CAD build for the part. Positions are in the model's coordinates, mm. A direction names the side the tool comes from. Give positions to 0.01 mm unless a question says otherwise; leave off trailing zeros. Write each loop counter-clockwise with the first axis right and the second up, starting at its lowest first coordinate (ties: lowest second). Pieces come first, ordered by that corner, then holes. Notation, with made-up numbers: (14.5, 22.25) - (70.5, 22.25) arc R18 ccw to (70.5, 50.25) - close; hole circle Ø10 at (79.5, -10). An arc over 180 degrees is marked (long way). Answer as a JSON object with one key per item and string values.
Autodesk Inventor part; units mm, degrees
ref_plane "YZ Plane" through (0, 0, 0) normal (1, 0, 0) x (0, 1, 0)
ref_plane "XZ Plane" through (0, 0, 0) normal (0, 1, 0) x (-1, 0, 0)
ref_plane "XY Plane" through (0, 0, 0) normal (0, 0, 1) x (1, 0, 0)
sketch "Sketch2" plane through (0, 0, 0) normal (0, 1, 0) x (-1, 0, 0)
  line L0 (0, 0) -> (85, 0)
  line L1 (85, 0) -> (85, -25)
  line L2 (85, -25) -> (0, -25)
  line L3 (0, -25) -> (0, 0)
  line L4 (-5, -25) -> (105, -25)
  line L5 (105, -25) -> (105, -40)
  line L6 (105, -40) -> (-5, -40)
  line L7 (-5, -40) -> (-5, -25)
  line L8 (-5, -25) -> (0, -20)
  dimension "d4" = 85
  dimension "d5" = 25
  dimension "d6" = 110
  dimension "d7" = 5
  dimension "d8" = 15
  dimension "d9" = 45
extrude "Extrusion2" add sketch "Sketch2" along normal blind 88
sketch "Sketch3" plane through (-105, 0, -25) normal (0, 0, 1) x (1, 0, 0)
  line L0 (20, 0) -> (20, 88)
  line L1 (20, 83) -> (1, 83)
  line L2 (1, 83) -> (1, 33)
  line L3 (1, 33) -> (20, 33)
  line L4 (20, 33) -> (20, 83)
  line L5 (0, 88) -> (20, 88)
  point P0 (105, 0)
  point P1 (20, 33)
  dimension "d12" = 50
  dimension "d13" = 19
  dimension "d14" = 5
extrude "Extrusion3" add sketch "Sketch3" along normal blind 15
sketch "Sketch4" plane through (-104, 33, -25) normal (-1, 0, 0) x (0, 0, 1)
  line L0 (6, 7.5) -> (11, 7.5)
  line L1 (11, 7.5) -> (11, 2.5)
  line L2 (11, 2.5) -> (6, 2.5)
  line L3 (6, 2.5) -> (6, 7.5)
  line L4 (0, -33) -> (0, 55)
  line L5 (0, 0) -> (15, 0)
  line L6 (6, 17.5) -> (11, 17.5)
  line L7 (11, 17.5) -> (11, 12.5)
  line L8 (6, 12.5) -> (6, 17.5)
  line L9 (11, 12.5) -> (6, 12.5)
  line L10 (6, 27.5) -> (11, 27.5)
  line L11 (11, 27.5) -> (11, 22.5)
  line L12 (6, 22.5) -> (6, 27.5)
  line L13 (11, 22.5) -> (6, 22.5)
  line L14 (6, 37.5) -> (11, 37.5)
  line L15 (11, 37.5) -> (11, 32.5)
  line L16 (6, 32.5) -> (6, 37.5)
  line L17 (11, 32.5) -> (6, 32.5)
  line L18 (6, 47.5) -> (11, 47.5)
  line L19 (11, 47.5) -> (11, 42.5)
  line L20 (6, 42.5) -> (6, 47.5)
  line L21 (11, 42.5) -> (6, 42.5)
  point P0 (25, -33)
  point P1 (6, 5)
  point P2 (7.5, 0)
  point P3 (8.5, 2.5)
  point P4 (6, 15)
  point P5 (8.5, 12.5)
  point P6 (6, 25)
  point P7 (8.5, 22.5)
  point P8 (6, 35)
  point P9 (8.5, 32.5)
  point P10 (6, 45)
  point P11 (8.5, 42.5)
  dimension "d17" = 6
  dimension "d18" = 5
  dimension "d19" = 2.5
  dimension "d20" = 5
  dimension "d23" = 10
extrude "Extrusion4" cut sketch "Sketch4" against normal blind 10
properties part number "PowerSupply"
(1) Pull direction Z, two halves, no side cores. Call faces 1 (the face through (-99, 75.5, -16)), 2 (the face through (-99, 68, -19)), 3 (the face through (-105, 43, -32)), 4 (the face through (-42, 43, 0)): pulls with the +Z half, pulls with the -Z half, needs draft (parallel to the pull), parting line crosses it, or undercut.
Answer key:
{"face 1": "undercut", "face 2": "undercut", "face 3": "needs draft", "face 4": "pulls with the +Z half"}
(2) Saw through at A-A, the plane y = 53. Give the cut face in (x, z).
Answer key:
{"outline": "(-105, -40) - (5, -40) - (5, -25) - (0, -20) - (0, 0) - (-85, 0) - (-85, -10) - (-104, -10) - (-104, -25) - (-105, -25) - close"}
(3) Probe L1, parallel to Y at x = -90.5, z = -21; L2, parallel to X at y = 72, z = -12.5; L3, parallel to X at y = 55.5, z = -2.5. List the from-to ranges inside material, lowest first. Write a range as [from, to].
Answer key:
{"L1": "y = [33, 83]", "L2": "x = [-104, 0]", "L3": "x = [-85, 0]"}
(4) 3-axis set-ups, long thin cutter, end or side, ignore diameter. For faces 5 (the face through (0, 43, -10)), 6 (the face through (-94, 83, -18)), 7 (the face through (-99, 58, -19)): which of +Z, -Z, +X, -X, +Y, -Y reach the whole face in a straight line?
Answer key:
{"face 5": "+Z, +X, +Y, -Y", "face 6": "+Z, -X, +Y", "face 7": "-X"}
(5) Flat gauge pins, fed straight in: P1, Ø1.5, axis at x = -100.5, y = 58.5, coming from the +Z side; P2, Ø4, axis at x = -98.5, z = -15.5, coming from the -Y side; P3, Ø4, axis at y = 27, z = -14.5, coming from the +X side. Where does each tip first touch, or does it go through?
Answer key:
{"P1": "stops at z = -10", "P2": "stops at y = 33", "P3": "stops at x = 0"}
